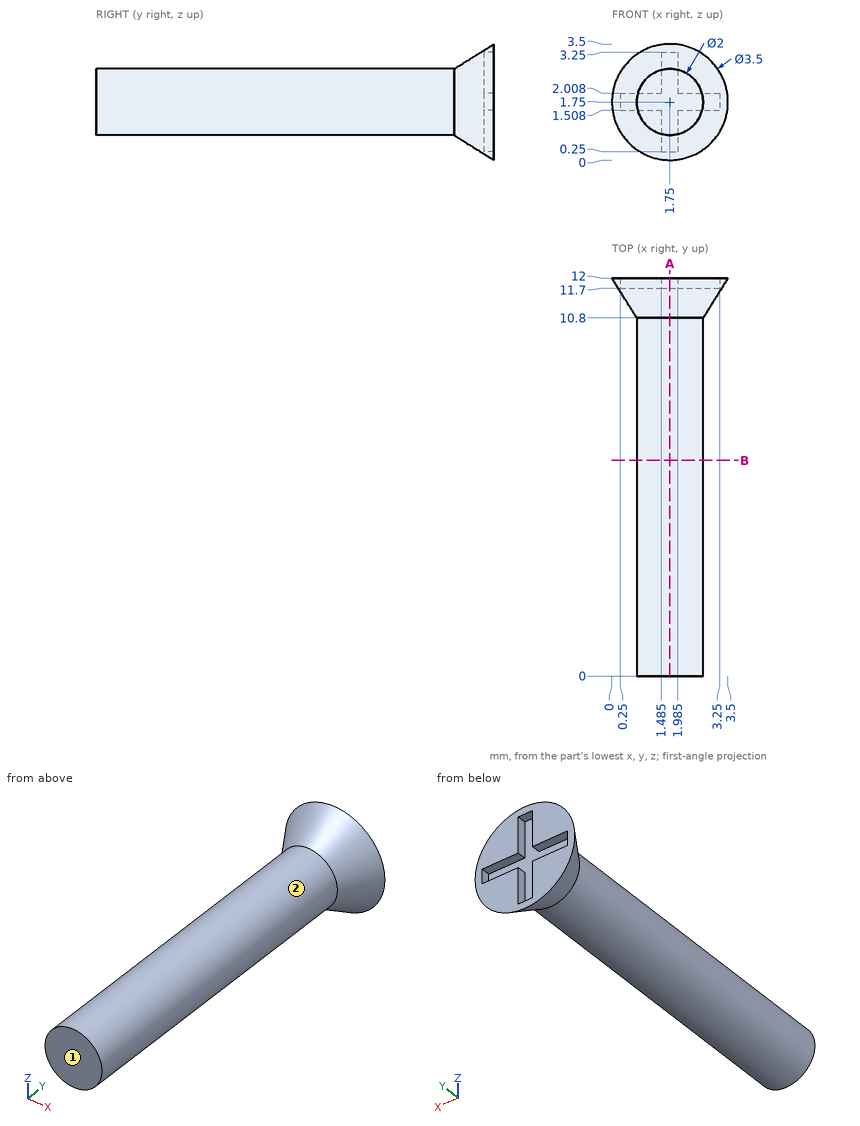
Design review of the part shown in the three views and the two pictorial views. Dimensions are in mm from the part's minimum x, y and z. A direction names the side the tool comes from. Give positions to 0.01 mm unless a question says otherwise; leave off trailing zeros. Loops run counter-clockwise (first coordinate to the right, second up) from the corner with the lowest first, then second, coordinate; pieces in that order, holes last. Notation, with made-up numbers: (32.25, 41) -> (77.25, 41) arc R22 cw to (77.25, 64) -> close; hole circle Ø10 at (-3, 43.5). An arc over 180 degrees is marked (long way). Write each question's results on one line, items separated by ' | '.
1) Tool access review of the marked faces 1 and 2: name each direction out of +Z, -Z, +X, -X, +Y, -Y from which nothing blocks a thin tool from reaching the whole face with its end or side.
Conclusion:
face 1: +Z, -Z, +X, -X, -Y | face 2: -Y
2) Insertion check: pin 1 Ø1 at (x, y) = (0.5, 4.5) entering from +Z; pin 2 Ø1 at (y, z) = (9, 2.5) entering from +X; pin 3 Ø1.5 at (x, y) = (1, 9.5) entering from -Z. Each pin has a flat end and moves straight along its axis. Give the tip position at first contact, or say it passes through.
Conclusion:
pin 1: stops at z = 2.41 | pin 2: stops at x = 2.72 | pin 3: stops at z = 0.75
3) Take a section at B-B, the plane y = 6.5. Give the boundary of the cut face in (x, z).
Conclusion:
outline: circle Ø2 at (1.75, 1.75)
4) For line 1 along Y through (x, z) = (1.55, 2); line 2 along Z through (x, y) = (1.7, 5.5); line 3 along X through (y, z) = (6, 1.55), list the stretches that pass through material, from the lowest coordinate up. Write a range as from..to.
Conclusion:
line 1: y = 0..11.7 | line 2: z = 0.75..2.75 | line 3: x = 0.77..2.73
5) Take a section at A-A, the plane x = 1.75. Give the boundary of the cut face in (y, z).
Conclusion:
outline: (0, 0.75) -> (10.8, 0.75) -> (12, 0) -> (12, 0.25) -> (11.7, 0.25) -> (11.7, 3.25) -> (12, 3.25) -> (12, 3.5) -> (10.8, 2.75) -> (0, 2.75) -> close
